Input: part model. Units: mm. Frame: model coordinates. A direction names the side the tool comes from. Round coordinates to 2 decimals unless told otherwise and drop trailing zeros. Order: outer loops, then holes, each group sorted by start corner. A loop starts at its lowest first (then second) coordinate and runs counter-clockwise, first axis right, second up. Notation, with made-up numbers: (83.25, 60.5) -> (97.25, 60.5) arc R19 cw to (97.25, 93.5) -> close; hole circle Ø6 at (22, 25). An arc over 180 degrees is marked (long way). Use a Markdown table: item, result.
from build123d import *

# Parameters (mm, degrees)
SKETCH1_R           = 7
SKETCH1_R_2         = 1.25
BOSS_EXTRUDE1_DEPTH = 17
SKETCH2_R           = 7
BOSS_EXTRUDE2_DEPTH = 11
SKETCH3_R           = 2.65
CUT_EXTRUDE1_DEPTH  = 2
SKETCH4_R           = 1.5
BOSS_EXTRUDE3_DEPTH = 5
SKETCH5_R           = 1.25
BOSS_EXTRUDE4_DEPTH = 5
SKETCH6_R           = 7
BOSS_EXTRUDE5_DEPTH = 15


with BuildPart() as part:
    # Sketch1 → Boss-Extrude1 (new body)
    with BuildSketch(Plane.XY):
        with Locations((-43.483141232, -69.989052064)):
            Circle(SKETCH1_R)
        with Locations((-43.483141232, -66.239052064)):
            Circle(SKETCH1_R_2, mode=Mode.SUBTRACT)
        with Locations((-40.235545968, -71.864052064)):
            Circle(SKETCH1_R_2, mode=Mode.SUBTRACT)
        with Locations((-46.730736496, -71.864052064)):
            Circle(SKETCH1_R_2, mode=Mode.SUBTRACT)
    extrude(amount=BOSS_EXTRUDE1_DEPTH)

    # Sketch2 → Boss-Extrude2 (add)
    with BuildSketch(Plane.XY.offset(17)):
        with Locations((-43.483141232, -69.989052064)):
            Circle(SKETCH2_R)
    extrude(amount=-BOSS_EXTRUDE2_DEPTH)

    # Sketch3 → Cut-Extrude1 (cut)
    with BuildSketch(Plane.XY.offset(17)):
        with Locations((-43.483141232, -69.989052064)):
            Circle(SKETCH3_R)
    extrude(amount=-CUT_EXTRUDE1_DEPTH, mode=Mode.SUBTRACT)

    # Sketch4 → Boss-Extrude3 (add)
    with BuildSketch(Plane(origin=(0, 0, 0), x_dir=(-1, 0, 0), z_dir=(0, 0, -1))):
        with Locations((43.483141232, -69.989052064)):
            Circle(SKETCH4_R)
    extrude(amount=BOSS_EXTRUDE3_DEPTH)

    # Sketch5 → Boss-Extrude4 (add, symmetric)
    with BuildSketch(Plane(origin=(0, 0, 0), x_dir=(-1, 0, 0), z_dir=(0, 0, -1))):
        with Locations((43.483141232, -66.239052064)):
            Circle(SKETCH5_R)
        with Locations((46.730736496, -71.864052064)):
            Circle(SKETCH5_R)
        with Locations((40.235545968, -71.864052064)):
            Circle(SKETCH5_R)
    extrude(amount=BOSS_EXTRUDE4_DEPTH, both=True)

    # Sketch6 → Boss-Extrude5 (add)
    with BuildSketch(Plane(origin=(0, 0, 0), x_dir=(-1, 0, 0), z_dir=(0, 0, -1))):
        with Locations((43.483141232, -69.989052064)):
            Circle(SKETCH6_R)
    extrude(amount=-BOSS_EXTRUDE5_DEPTH)


solid = part.part
1) Set-up query: faces 1 (the face through (-44, -68, 0)), 2 (the face through (-44, -70, 15)), 3 (the face through (-43, -70, -5)). Return all of +Z, -Z, +X, -X, +Y, -Y with unobstructed straight access to the full face (end or side cutting, diameter ignored); none if empty.
Answer key:
| item | result |
|---|---|
| face 1 | -Z |
| face 2 | +Z |
| face 3 | -Z, +X, -X, +Y, -Y |
2) Cut plane C-C on y = -69.75. Return loops of the section in (x, z).
Answer key:
| item | result |
|---|---|
| outline | (-50.48, 0) -> (-44.96, 0) -> (-44.96, -5) -> (-42, -5) -> (-42, 0) -> (-36.49, 0) -> (-36.49, 17) -> (-40.84, 17) -> (-40.84, 15) -> (-46.12, 15) -> (-46.12, 17) -> (-50.48, 17) -> close |
3) Cut plane D-D on z = 10. Return loops of the section in (x, y), and give its area (3 significant figures).
Answer key:
| item | result |
|---|---|
| outline | circle Ø14 at (-43.48, -69.99) |
| area | 154 mm^2 |
4) Draft query along Y for faces 4 (the face through (-42.234, -66.184, -2.465)), 5 (the face through (-42.378, -68.975, -2.465)), 6 (the face through (-39.7, -64.1, 8.4)), 7 (the face through (-47, -72, -5)). Return one class per face: released by +Y, released by -Y, zero draft, split by the parting line, or undercut.
Answer key:
| item | result |
|---|---|
| face 4 | undercut |
| face 5 | undercut |
| face 6 | split by the parting line |
| face 7 | zero draft |
5) Ray query, probe 1 along Z at (x, y) = (-44.5, -69.75); probe 2 along Z at (x, y) = (-36.75, -69.25); probe 3 along X at (y, z) = (-72, 14.75). Return the intervals inside material, ascending.
Answer key:
| item | result |
|---|---|
| probe 1 | z = -5 to 15 |
| probe 2 | z = 0 to 17 |
| probe 3 | x = -50.19 to -36.78 |
6) Contact query for flat-ended pins moving along their axis: P1, Ø2.5, axis at x = -43, y = -71, coming from the +Z side; P2, Ø5, axis at y = -67, z = 6.5, coming from the +X side; P3, Ø3, axis at y = -66, z = 14, coming from the -X side. Output: stop coordinate, or through.
Answer key:
| item | result |
|---|---|
| P1 | stops at z = 15 |
| P2 | stops at x = -36.5 |
| P3 | stops at x = -50.03 |
7) Cut plane B-B on z = -0.5. Return loops of the section in (x, y).
Answer key:
| item | result |
|---|---|
| outline | circle Ø2.5 at (-46.73, -71.86); circle Ø3 at (-43.48, -69.99); circle Ø2.5 at (-43.48, -66.24); circle Ø2.5 at (-40.24, -71.86) |
8) Cut plane A-A on x = -39.5. Return loops of the section in (y, z).
Answer key:
| item | result |
|---|---|
| outline | (-75.75, 0) -> (-72.87, 0) -> (-72.87, -5) -> (-70.85, -5) -> (-70.85, 0) -> (-64.23, 0) -> (-64.23, 17) -> (-75.75, 17) -> close |
